```python
from build123d import *

# Parameters (mm, degrees)
ESQUISSE1_R        = 0.75
ESQUISSE1_R_2      = 1
BOSS_EXTRU_1_DEPTH = 2
ESQUISSE2_R        = 3.75
ESQUISSE2_R_2      = 2
BOSS_EXTRU_2_DEPTH = 3


with BuildPart() as part:
    # Esquisse1 → Boss.-Extru.1 (new body)
    with BuildSketch(Plane(origin=(0, 0, 0), x_dir=(1, 0, 0), z_dir=(0, 1, 0))):
        with BuildLine():
            Line((0, 4), (16, 2.5))
            ThreePointArc((16, 2.5), (18.5, 0), (16, -2.5))
            Line((16, -2.5), (0, -4))
            ThreePointArc((0, -4), (-4, 0), (0, 4))
        make_face()
        with Locations(Location((16, 0, 0), (0, 0, 270))):
            Circle(ESQUISSE1_R, mode=Mode.SUBTRACT)
        with Locations(Location((13, 0, 0), (0, 0, 270))):
            Circle(ESQUISSE1_R, mode=Mode.SUBTRACT)
        with Locations(Location((10, 0, 0), (0, 0, 270))):
            Circle(ESQUISSE1_R, mode=Mode.SUBTRACT)
        with Locations(Location((7, 0, 0), (0, 0, 270))):
            Circle(ESQUISSE1_R, mode=Mode.SUBTRACT)
        with Locations(Location((0, 0, 0), (0, 0, 270))):
            Circle(ESQUISSE1_R_2, mode=Mode.SUBTRACT)
    extrude(amount=BOSS_EXTRU_1_DEPTH)

    # Esquisse2 → Boss.-Extru.2 (add)
    with BuildSketch(Plane(origin=(0, 2, 0), x_dir=(1, 0, 0), z_dir=(0, 1, 0))):
        with Locations(Location((0, 0, 0), (0, 0, 270))):
            Circle(ESQUISSE2_R)
        with Locations(Location((0, 0, 0), (0, 0, 270))):
            Circle(ESQUISSE2_R_2, mode=Mode.SUBTRACT)
    extrude(amount=BOSS_EXTRU_2_DEPTH)


solid = part.part
```
The model under review builds one solid part; all positions refer to its coordinate system, in mm. A direction names the side the tool comes from. Round coordinates to 2 decimals unless told otherwise and drop trailing zeros. Write each loop counter-clockwise with the first axis right and the second up, starting at its lowest first coordinate (ties: lowest second). Pieces come first, ordered by that corner, then holes. Notation, with made-up numbers: (74, 43) - (123, 43) arc R30 cw to (123, 77) - close; hole circle Ø8 at (-22.75, 3.5). An arc over 180 degrees is marked (long way). Answer as CSV lines item,"result". Start each with the question number.
(1) For pin 1 Ø1.5 at (y, z) = (1, -1.5) entering from -X; pin 2 Ø1.2 at (x, z) = (16, 0) entering from -Y; pin 3 Ø1 at (y, z) = (1.5, -2) entering from -X; pin 4 Ø1.5 at (y, z) = (1.5, -3) entering from -X, all flat-tipped, find the tip position at first contact; note any pin that passes through.
(2) For faces 1 (the cylindrical face through (13.744, 0.986, -0.098)), 2 (the flat face through (-1, 2, 1)), list the 3-axis set-ups (+Z, -Z, +X, -X, +Y, -Y) from which the entire face can be reached by the end or side of a thin tool; tool diameter is ignored.
(3) We need section B-B on y = 0.7. State the section outline as (x, z) points.
(4) We need section C-C on x = 7. State the section outline as (y, z) points, plus the area to 3 significant figures.
(5) We need section D-D on y = 2.35. State the section outline as (x, z) points.
(6) We need section A-A on z = 0. Give the number of separate pieces and of enclosed holes in the cut face, plus the area to 3 significant figures.
(7) To check wall thickness, follow line 1 (X direction, y = 0.5, z = 0); line 2 (Y direction, x = 2.5, z = 3.25); line 3 (Z direction, x = 13.5, y = 1.75). State the ranges of each line that lie inside material, in increasing order.
(8) Draft analysis for pull direction Z (two halves, no side actions). For faces 3 (the cylindrical face through (-4, 1, 0)), 4 (the cylindrical face through (7.225, 0.986, 0.715)), 5 (the flat face through (7.89, 0.99, -3.26)), state which applies: pulls with the +Z half, pulls with the -Z half, needs draft (parallel to the pull), parting line crosses it, or undercut.
Worked answers:
1,pin 1,"x = -3.93"
1,pin 2,"through"
1,pin 3,"x = -3.71"
1,pin 4,"x = -3.31"
2,face 1,"+Y, -Y"
2,face 2,"+Y"
3,outline,"(0, -4) - (16, -2.5) arc R2.5 ccw to (16, 2.5) - (0, 4) arc R4 ccw to start; hole circle Ø2 at (0, 0); hole circle Ø1.5 at (7, 0); hole circle Ø1.5 at (10, 0); hole circle Ø1.5 at (13, 0); hole circle Ø1.5 at (16, 0)"
4,outline,"(0, -3.34) - (2, -3.34) - (2, -0.75) - (0, -0.75) - close; (0, 0.75) - (2, 0.75) - (2, 3.34) - (0, 3.34) - close"
4,area,"10.4 mm²"
5,outline,"circle Ø7.5 at (0, 0); hole circle Ø4 at (0, 0)"
6,separate pieces,"6"
6,enclosed holes,"0"
6,area,"39.5 mm²"
7,line 1,"-4 to -1, 1 to 6.25, 7.75 to 9.25, 10.75 to 12.25, 13.75 to 15.25, 16.75 to 18.5"
7,line 2,"0 to 2"
7,line 3,"-2.73 to -0.56, 0.56 to 2.73"
8,face 3,"parting line crosses it"
8,face 4,"undercut"
8,face 5,"pulls with the -Z half"
